from build123d import *

# Parameters (mm, degrees)
SKETCH1_W                     = 12
SKETCH1_H                     = 12
BOSS_EXTRUDE1_DEPTH           = 5.03
TAP_DRILL_FOR_0_80_TAP1_D     = 1.19126
TAP_DRILL_FOR_0_80_TAP1_DEPTH = 4
TAP_DRILL_FOR_0_80_TAP1_TIP   = 0.357890611
F_2_CLEARANCE_HOLE1_D         = 2.4384


with BuildPart() as part:
    # Sketch1 → Boss-Extrude1 (new body)
    with BuildSketch(Plane(origin=(0, 0, 0), x_dir=(0, 0, -1), z_dir=(1, 0, 0))):
        with Locations((6, 6)):
            Rectangle(SKETCH1_W, SKETCH1_H)
    extrude(amount=BOSS_EXTRUDE1_DEPTH)

    # Tap Drill for #0-80 Tap1
    with Locations(Plane.XY):
        with Locations((2.515, 9.5)):
            Hole(TAP_DRILL_FOR_0_80_TAP1_D / 2, depth=TAP_DRILL_FOR_0_80_TAP1_DEPTH)
            with Locations((0, 0, -(TAP_DRILL_FOR_0_80_TAP1_DEPTH + TAP_DRILL_FOR_0_80_TAP1_TIP / 2))):  # 118° drill point
                Cone(0, TAP_DRILL_FOR_0_80_TAP1_D / 2, TAP_DRILL_FOR_0_80_TAP1_TIP, mode=Mode.SUBTRACT)

    # #2 Clearance Hole1 (through all)
    with Locations(Plane(origin=(5.03, 0, 0), x_dir=(0, 0, -1), z_dir=(1, 0, 0))):
        with Locations((7.5, 6.5)):
            Hole(F_2_CLEARANCE_HOLE1_D / 2)


solid = part.part
Read the model definition and answer for the solid it produces. Units are mm, in the model's axes. Coordinates: 2 decimals unless noted, no trailing zeros. Loops run counter-clockwise (first coordinate to the right, second up) from the corner with the lowest first, then second, coordinate; pieces in that order, holes last. Notation, with made-up numbers: (31, 13) - (78, 13) arc R23 cw to (78, 52) - close; hole circle Ø8 at (36.5, 78.25). An arc over 180 degrees is marked (long way). Answer in a Markdown table with one row per item.
Q1. Given P1, Ø1, axis at x = 3, z = -8.5, coming from the -Y side, flat-ended and moving along its own axis, determine where the tip first touches the part or whether it passes through.
Here are the results:
| item | result |
|---|---|
| P1 | stops at y = 0 |
Q2. Find section A-A on z = -7.5. Write down the section's boundary in (x, y).
Here are the results:
| item | result |
|---|---|
| outline | (0, 0) - (5.03, 0) - (5.03, 5.28) - (0, 5.28) - close; (0, 7.72) - (5.03, 7.72) - (5.03, 12) - (0, 12) - close |
Q3. The mould has two halves that part along Y. Classify faces 1 (the cylindrical face through (2.644, 8.919, -2.028)), 2 (the flat face through (2, 0, -6)), 3 (the flat face through (2, 12, -6)): pulls with the +Y half, pulls with the -Y half, needs draft (parallel to the pull), parting line crosses it, or undercut.
Here are the results:
| item | result |
|---|---|
| face 1 | undercut |
| face 2 | pulls with the -Y half |
| face 3 | pulls with the +Y half |
Q4. Find section B-B on y = 6.5. Write down the section's boundary in (x, z).
Here are the results:
| item | result |
|---|---|
| outline | (0, -12) - (5.03, -12) - (5.03, -8.72) - (0, -8.72) - close; (0, -6.28) - (5.03, -6.28) - (5.03, 0) - (0, 0) - close |
Q5. Find section C-C on z = -2. Write down the section's boundary in (x, y) (3 decimals), plus the area to 3 significant figures.
Here are the results:
| item | result |
|---|---|
| outline | (0, 0) - (5.03, 0) - (5.03, 12) - (0, 12) - close; hole circle Ø1.191 at (2.515, 9.5) |
| area | 59.2 mm^2 |
Q6. Straight lines are drawn through the part: line 1 along Y through (x, z) = (1.6, -7.5); line 2 along X through (y, z) = (9.5, -2.9); line 3 along Y through (x, z) = (2.8, -1.5). For each, find the intervals that lie inside material, in ascending order. Write a range as [from, to].
Here are the results:
| item | result |
|---|---|
| line 1 | y = [0, 5.28], [7.72, 12] |
| line 2 | x = [0, 1.92], [3.11, 5.03] |
| line 3 | y = [0, 8.98], [10.02, 12] |
